```python
from build123d import *

# Parameters (mm, degrees)
SKETCH1_R           = 19.05
BOSS_EXTRUDE1_DEPTH = 6.35
SKETCH2_W           = 12.7
SKETCH2_H           = 50.8
BOSS_EXTRUDE4_DEPTH = 25.4


with BuildPart() as part:
    # Sketch1 → Boss-Extrude1 (new body)
    with BuildSketch(Plane(origin=(0, 0, 0), x_dir=(1, 0, 0), z_dir=(0, 1, 0))):
        with BuildLine():
            Line((-38.1, 0), (-38.1, -177.8))
            ThreePointArc((-38.1, -177.8), (0, -215.9), (38.1, -177.8))
            Line((38.1, -177.8), (38.1, 0))
            ThreePointArc((38.1, 0), (0, 38.1), (-38.1, 0))
        make_face()
        with Locations(Location((0, 0, 0), (0, 0, 270))):
            Circle(SKETCH1_R, mode=Mode.SUBTRACT)
        with Locations(Location((0, -177.8, 0), (0, 0, 270))):
            Circle(SKETCH1_R, mode=Mode.SUBTRACT)
    extrude(amount=BOSS_EXTRUDE1_DEPTH)

    # Sketch2 → Boss-Extrude4 (add)
    with BuildSketch(Plane(origin=(0, 6.35, 0), x_dir=(1, 0, 0), z_dir=(0, 1, 0))):
        with Locations((-44.45, -63.5)):
            Rectangle(SKETCH2_W, SKETCH2_H)
    extrude(amount=-BOSS_EXTRUDE4_DEPTH)


solid = part.part
```
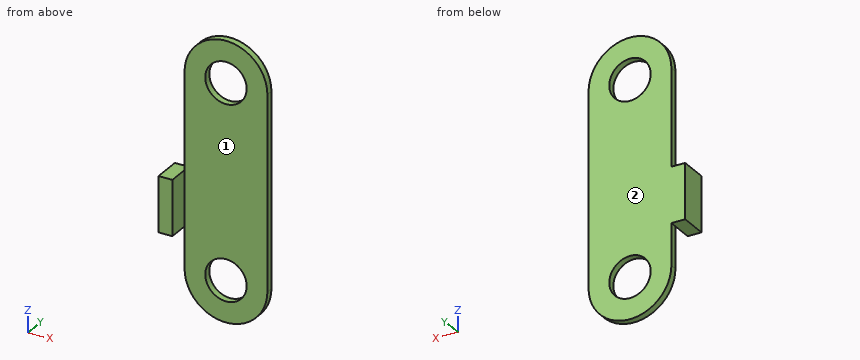
Design review of the part built by this model. Coordinates are the model's own, in mm. Face numbers are marked on the shaded views. A direction names the side the tool comes from. Give positions to 0.01 mm unless a question says otherwise; leave off trailing zeros. Write each loop counter-clockwise with the first axis right and the second up, starting at its lowest first coordinate (ties: lowest second). Pieces come first, ordered by that corner, then holes. Notation, with made-up numbers: (-19.75, 76) - (7.25, 76) arc R31 cw to (7.25, 105) - close; hole circle Ø10 at (50.25, -14). An arc over 180 degrees is marked (long way). Return JSON: item names as keys, results as strings. Group by question number.
(1) Insertion check: pin 1 (4 mm diameter, centred on y = -3, z = 74, fed in from +X); pin 2 (6.5 mm diameter, centred on x = -44.5, y = -6, fed in from +Z); pin 3 (5 mm diameter, centred on y = 3.5, z = 17.5, fed in from -X). Each pin has a flat end and moves straight along its axis. Give the tip position at first contact, or say it passes through.
(2) We need section A-A, the plane x = 0. Give the boundary of the cut face in (y, z), then the cut area to 3 significant figures.
(3) We need section C-C, the plane z = 66. Give the boundary of the cut face in (x, y), then the cut area to 3 significant figures.
(4) We need section D-D, the plane y = -7.5. Give the boundary of the cut face in (x, z), then the cut area to 3 significant figures.
(5) Machinability: for the marked faces 1 and 2, which of the approach directions +Z, -Z, +X, -X, +Y, -Y give a long, thin tool a straight path to every point of the face, cutting with its end or side? Answer none if there is none.
(6) To check wall thickness, follow probe 1 along X at (y, z) = (2, 177.8); probe 2 along X at (y, z) = (0.75, 98); probe 3 along Y at (x, z) = (-5, 85.5). State the ranges of each line that lie inside material, in increasing order.
(7) We need section B-B, the plane z = 3. Give the boundary of the cut face in (x, y), then the cut area to 3 significant figures.
Reported:
{
 "1": {"pin 1": "stops at x = -38.1", "pin 2": "stops at z = 88.9", "pin 3": "stops at x = -38.1"},
 "2": {"outline": "(0, -38.1) - (6.35, -38.1) - (6.35, -19.05) - (0, -19.05) - close; (0, 19.05) - (6.35, 19.05) - (6.35, 158.75) - (0, 158.75) - close; (0, 196.85) - (6.35, 196.85) - (6.35, 215.9) - (0, 215.9) - close", "area": "1,130 mm2"},
 "3": {"outline": "(-50.8, -19.05) - (-38.1, -19.05) - (-38.1, 0) - (38.1, 0) - (38.1, 6.35) - (-50.8, 6.35) - close", "area": "806 mm2"},
 "4": {"outline": "(-50.8, 38.1) - (-38.1, 38.1) - (-38.1, 88.9) - (-50.8, 88.9) - close", "area": "645 mm2"},
 "5": {"face 1": "+Z, -Z, +X, -Y", "face 2": "+Z, -Z, +X, -X, +Y"},
 "6": {"probe 1": "x = -38.1 to -19.05, 19.05 to 38.1", "probe 2": "x = -38.1 to 38.1", "probe 3": "y = 0 to 6.35"},
 "7": {"outline": "(-38.1, 0) - (-18.81, 0) - (-18.81, 6.35) - (-38.1, 6.35) - close; (18.81, 0) - (38.1, 0) - (38.1, 6.35) - (18.81, 6.35) - close", "area": "245 mm2"}
}
